For this review, take the finished solid that the model builds, in its own axes (mm). Face numbers are marked on the shaded views. A direction names the side the tool comes from. Coordinates: 2 decimals unless noted, no trailing zeros. Loops run counter-clockwise (first coordinate to the right, second up) from the corner with the lowest first, then second, coordinate; pieces in that order, holes last. Notation, with made-up numbers: (54.25, 5) -> (80.25, 5) arc R21 cw to (80.25, 17) -> close; hole circle Ø4 at (72.25, -36.75). An arc over 180 degrees is marked (long way). Use a Markdown table: item, result.
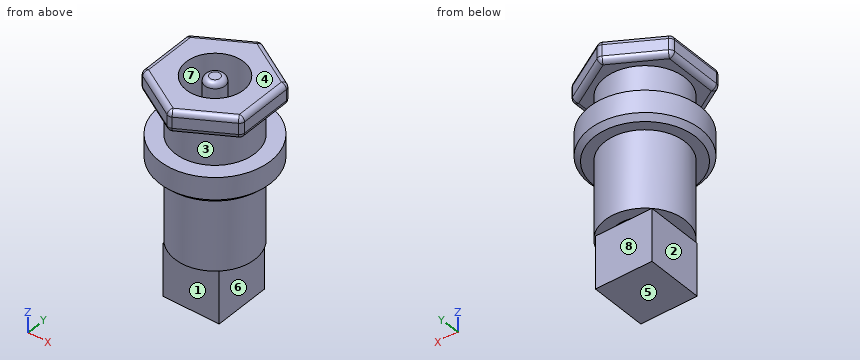
Autodesk Inventor part; units mm, degrees
ref_plane "YZ Plane" through (0, 0, 0) normal (1, 0, 0) x (0, 1, 0)
ref_plane "XZ Plane" through (0, 0, 0) normal (0, 1, 0) x (-1, 0, 0)
ref_plane "XY Plane" through (0, 0, 0) normal (0, 0, 1) x (1, 0, 0)
sketch "Sketch1" plane through (0, 0, 0) normal (0, 0, 1) x (1, 0, 0)
  circle A0 centre (0, 0) radius 5.5
  circle A1 centre (0, 0) radius 1
  circle A2 centre (0, 0) radius 3.9688
  circle A3 centre (0, 0) radius 2.85
  dimension "d0" = 11
  dimension "d1" = 2
  dimension "d2" = 7.9375
  dimension "d3" = 5.7
extrude "Extrusion1" add sketch "Sketch1" along normal blind 5.7 and the other way blind 10.4 contours A2
extrude "Extrusion2" add sketch "Sketch1" against normal blind 2.7 contours A0
extrude "Extrusion3" add sketch "Sketch1" along normal blind 5.7 contours A1
extrude "Extrusion4" add sketch "Sketch1" against normal blind 2.7 contours A1 | A2 | A3
sketch "Sketch2" plane through (0, 0, -10.4) normal (0, 0, -1) x (-1, 0, 0)
  circle A0 centre (0, 0) radius 3.9688
  line L0 (2.8725, 2.7386) -> (-2.7241, 2.7386)
  line L1 (-2.7241, 2.7386) -> (-2.7241, -2.8862)
  line L2 (-2.7241, -2.8862) -> (2.8725, -2.8862)
  line L3 (2.8725, -2.8862) -> (2.8725, 2.7386)
extrude "Extrusion5" add sketch "Sketch2" along normal blind 5.2 contours L3 A0 L2 L1 L0 | L3 L2 A0
sketch "Sketch3" plane through (0, 0, 5.7) normal (0, 0, 1) x (1, 0, 0)
  line L0 (5, -2.8868) -> (5, 2.8868)
  line L1 (0, 5.7735) -> (5, 2.8868)
  line L2 (0, 5.7735) -> (-5, 2.8868)
  line L3 (-5, 2.8868) -> (-5, -2.8868)
  line L4 (-5, -2.8868) -> (0, -5.7735)
  line L5 (0, -5.7735) -> (5, -2.8868)
  circle A0 centre (0, 0) radius 3.9688
extrude "Extrusion6" add sketch "Sketch3" against normal blind 2.1
fillet "Fillet1" radius 0.5 18 edges at (-2.5, -4.3301, 5.7) (2.5, -4.3301, 5.7) (2.5, -4.3301, 3.6) (-2.5, -4.3301, 3.6) (-5, 0, 3.6) (-5, 0, 5.7) (5, 0, 5.7) (2.5, 4.3301, 5.7) (-2.5, 4.3301, 5.7) (0, -5.7735, 4.65) (5, -2.8868, 4.65) (-5, -2.8868, 4.65) (-5, 2.8868, 4.65) (-2.5, 4.3301, 3.6) (0, 5.7735, 4.65) (2.5, 4.3301, 3.6) (5, 2.8868, 4.65) (5, 0, 3.6)
fillet "Fillet2" radius 0.5 1 edges at (-1, 0, 5.7)
chamfer "Chamfer1" distance 0.5 angle 45 1 edges at (-5.5, 0, -2.7)
thread "Thread1"
properties part number "Power_Socket"
(1) Take a section at C-C on z = -1. Write out the cut boundary in (x, y).
Found:
| item | result |
|---|---|
| outline | circle Ø11 at (0, 0) |
(2) For line 1 along Y through (x, z) = (0, 2.6); line 2 along Z through (x, y) = (0.75, -0.5); line 3 along Z through (x, y) = (-3.75, -1.5), list the stretches that pass through material, from the lowest coordinate up.
Found:
| item | result |
|---|---|
| line 1 | y = -3.97 to -2.85, -1 to 1, 2.85 to 3.97 |
| line 2 | z = -15.6 to -10.4, -2.7 to 5.5 |
| line 3 | z = -2.7 to 0, 3.6 to 5.7 |
(3) For the marked faces 1, 2, 3, 4 and 5, list the 3-axis set-ups (+Z, -Z, +X, -X, +Y, -Y) from which the entire face can be reached by the end or side of a thin tool; tool diameter is ignored.
Found:
| item | result |
|---|---|
| face 1 | -Z, +X, -X, -Y |
| face 2 | -Z, -X, +Y, -Y |
| face 3 | none |
| face 4 | +Z, +X, -X, +Y, -Y |
| face 5 | -Z, +X, -X, +Y, -Y |
(4) Take a section at B-B on z = -6.5. Write out the cut boundary in (x, y), plus the area to 3 significant figures.
Found:
| item | result |
|---|---|
| outline | circle Ø7.94 at (0, 0); hole circle Ø5.7 at (0, 0) |
| area | 24.0 mm^2 |
(5) Take a section at A-A on z = 1.25. Write out the cut boundary in (x, y).
Found:
| item | result |
|---|---|
| outline | circle Ø7.94 at (0, 0); circle Ø2 at (0, 0); hole circle Ø5.7 at (0, 0) |
(6) Mouldability with a two-part tool opening along X and no side actions: class the marked faces 6, 7 and 8 as pulls with the +X half, pulls with the -X half, needs draft (parallel to the pull), parting line crosses it, or undercut.
Found:
| item | result |
|---|---|
| face 6 | pulls with the +X half |
| face 7 | undercut |
| face 8 | needs draft |
(7) For pin 1 Ø4 at (x, z) = (0.5, -1) entering from -Y; pin 2 Ø2 at (x, z) = (3.5, -12) entering from -Y; pin 3 Ø4 at (x, z) = (-2.5, -10.5) entering from -Y, all flat-tipped, find the tip position at first contact; note any pin that passes through.
Found:
| item | result |
|---|---|
| pin 1 | stops at y = -5.5 |
| pin 2 | stops at y = -2.89 |
| pin 3 | stops at y = -3.94 |
